Check sheet for the modelled part. Datum: model origin and axes. Units: mm. Give positions to 0.01 mm unless a question says otherwise; leave off trailing zeros. Order: outer loops, then holes, each group sorted by start corner. A loop starts at its lowest first (then second) coordinate and runs counter-clockwise, first axis right, second up.
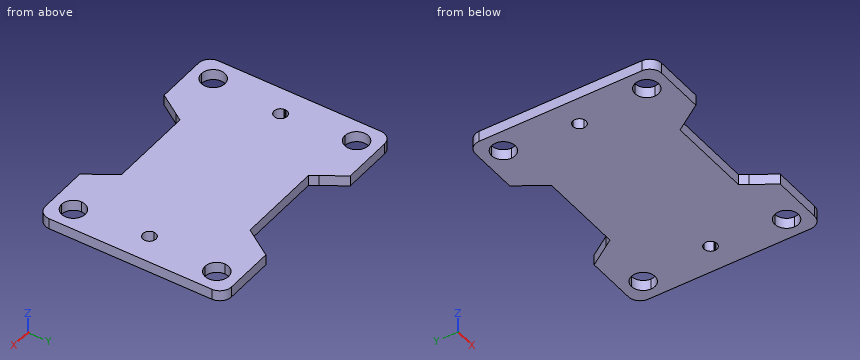
```python
from build123d import *

# Parameters (mm, degrees)
BOSS_EXTRUDE1_DEPTH = 2.5
FILLET1_R           = 2.75


with BuildPart() as part:
    # Sketch1 → Boss-Extrude1 (new body)
    with BuildSketch(Plane.XY):
        with BuildLine():
            ThreePointArc((0, 16.504235885), (-0.014991749, 16.62671172), (-0.02, 16.75))
            Line((-0.02, 16.75), (-5, 16.75))
            Line((-5, 16.75), (-5, -5))
            Line((-5, -5), (9.5, -5))
            Line((9.5, -5), (12.833333333, 0))
            Line((12.833333333, 0), (2.75, 0))
            ThreePointArc((2.75, 0), (1.944543648, -1.944543648), (0, -2.75))
            ThreePointArc((0, -2.75), (-2.75, 0), (0, 2.75))
            Line((0, 2.75), (0, 16.504235885))
        make_face()
        with BuildLine():
            ThreePointArc((0, 30.75), (-2.75, 33.5), (0, 36.25))
            ThreePointArc((0, 36.25), (1.944543648, 35.444543648), (2.75, 33.5))
            Line((2.75, 33.5), (12.833333333, 33.5))
            Line((12.833333333, 33.5), (9.5, 38.5))
            Line((9.5, 38.5), (-5, 38.5))
            Line((-5, 38.5), (-5, 16.75))
            Line((-5, 16.75), (-0.02, 16.75))
            ThreePointArc((-0.02, 16.75), (-0.014991749, 16.87328828), (0, 16.995764115))
            Line((0, 16.995764115), (0, 30.75))
        make_face()
        with BuildLine():
            ThreePointArc((2.75, 33.5), (1.944543648, 31.555456352), (0, 30.75))
            Line((0, 30.75), (0, 16.995764115))
            ThreePointArc((0, 16.995764115), (0.51591704, 17.908438918), (1.5, 18.27))
            ThreePointArc((1.5, 18.27), (2.574802307, 17.824802307), (3.02, 16.75))
            Line((3.02, 16.75), (24, 16.75))
            Line((24, 16.75), (24, 31.75))
            Line((24, 31.75), (14, 31.75))
            Line((14, 31.75), (12.833333333, 33.5))
            Line((12.833333333, 33.5), (2.75, 33.5))
        make_face()
        with BuildLine():
            Line((45.25, 33.5), (35.166666667, 33.5))
            Line((35.166666667, 33.5), (34, 31.75))
            Line((34, 31.75), (24, 31.75))
            Line((24, 31.75), (24, 16.75))
            Line((24, 16.75), (44.98, 16.75))
            ThreePointArc((44.98, 16.75), (45.425197693, 17.824802307), (46.5, 18.27))
            ThreePointArc((46.5, 18.27), (47.48408296, 17.908438918), (48, 16.995764115))
            Line((48, 16.995764115), (48, 30.75))
            ThreePointArc((48, 30.75), (46.055456352, 31.555456352), (45.25, 33.5))
        make_face()
        with BuildLine():
            Line((38.5, 38.5), (35.166666667, 33.5))
            Line((35.166666667, 33.5), (45.25, 33.5))
            ThreePointArc((45.25, 33.5), (46.055456352, 35.444543648), (48, 36.25))
            ThreePointArc((48, 36.25), (49.944543648, 35.444543648), (50.75, 33.5))
            ThreePointArc((50.75, 33.5), (49.944543648, 31.555456352), (48, 30.75))
            Line((48, 30.75), (48, 16.995764115))
            ThreePointArc((48, 16.995764115), (48.014991749, 16.87328828), (48.02, 16.75))
            Line((48.02, 16.75), (53, 16.75))
            Line((53, 16.75), (53, 38.5))
            Line((53, 38.5), (38.5, 38.5))
        make_face()
        with BuildLine():
            ThreePointArc((48.02, 16.75), (48.014991749, 16.62671172), (48, 16.504235885))
            Line((48, 16.504235885), (48, 2.75))
            ThreePointArc((48, 2.75), (49.944543648, 1.944543648), (50.75, 0))
            ThreePointArc((50.75, 0), (49.944543648, -1.944543648), (48, -2.75))
            ThreePointArc((48, -2.75), (46.055456352, -1.944543648), (45.25, 0))
            Line((45.25, 0), (35.166666667, 0))
            Line((35.166666667, 0), (38.5, -5))
            Line((38.5, -5), (53, -5))
            Line((53, -5), (53, 16.75))
            Line((53, 16.75), (48.02, 16.75))
        make_face()
        with BuildLine():
            Line((44.98, 16.75), (24, 16.75))
            Line((24, 16.75), (24, 1.75))
            Line((24, 1.75), (34, 1.75))
            Line((34, 1.75), (35.166666667, 0))
            Line((35.166666667, 0), (45.25, 0))
            ThreePointArc((45.25, 0), (46.055456352, 1.944543648), (48, 2.75))
            Line((48, 2.75), (48, 16.504235885))
            ThreePointArc((48, 16.504235885), (46.37671172, 15.235008251), (44.98, 16.75))
        make_face()
        with BuildLine():
            ThreePointArc((3.02, 16.75), (1.62328828, 15.235008251), (0, 16.504235885))
            Line((0, 16.504235885), (0, 2.75))
            ThreePointArc((0, 2.75), (1.944543648, 1.944543648), (2.75, 0))
            Line((2.75, 0), (12.833333333, 0))
            Line((12.833333333, 0), (14, 1.75))
            Line((14, 1.75), (24, 1.75))
            Line((24, 1.75), (24, 16.75))
            Line((24, 16.75), (3.02, 16.75))
        make_face()
    extrude(amount=BOSS_EXTRUDE1_DEPTH)

    # Fillet1
    fillet1_edges = [part.edges().sort_by_distance(p)[0] for p in [
        (53, -5, 1.25),
        (-5, -5, 1.25),
        (-5, 38.5, 1.25),
        (53, 38.5, 1.25),
    ]]
    fillet(fillet1_edges, radius=FILLET1_R)


solid = part.part
```
(1) Material ranges on L1, parallel to Y at x = 47.5, z = 0.9; L2, parallel to X at y = 18, z = 0.3; L3, parallel to X at y = 32, z = 0.3, recorded low to high.
Response values:
L1: y = -5 to -2.7, 2.7 to 15.61, 17.89 to 30.8, 36.2 to 38.5
L2: x = -5 to 0.64, 2.36 to 45.64, 47.36 to 53
L3: x = -5 to -2.3, 2.3 to 13.83, 34.17 to 45.7, 50.3 to 53
(2) Cross-section at C-C on z = 0.5. Enter the section's corners in (x, y), then the cut area to 3 significant figures.
Response values:
outline: (-5, -2.25) arc R2.75 ccw to (-2.25, -5) - (9.5, -5) - (14, 1.75) - (34, 1.75) - (38.5, -5) - (50.25, -5) arc R2.75 ccw to (53, -2.25) - (53, 35.75) arc R2.75 ccw to (50.25, 38.5) - (38.5, 38.5) - (34, 31.75) - (14, 31.75) - (9.5, 38.5) - (-2.25, 38.5) arc R2.75 ccw to (-5, 35.75) - close; hole circle Ø5.5 at (0, 0); hole circle Ø5.5 at (0, 33.5); hole circle Ø3.04 at (1.5, 16.75); hole circle Ø3.04 at (46.5, 16.75); hole circle Ø5.5 at (48, 0); hole circle Ø5.5 at (48, 33.5)
area: 2,080 mm2
(3) Gauge pin test, flat end, axial feed: pin 1 Ø1.2 at (x, z) = (23.5, 0.5) entering from -Y. Record the tip position at first contact, or that the pin passes through.
Response values:
pin 1: stops at y = 1.75
(4) Cross-section at A-A on x = 49. Enter the section's corners in (y, z).
Response values:
outline: (-5, 0) - (-2.56, 0) - (-2.56, 2.5) - (-5, 2.5) - close; (2.56, 0) - (30.94, 0) - (30.94, 2.5) - (2.56, 2.5) - close; (36.06, 0) - (38.5, 0) - (38.5, 2.5) - (36.06, 2.5) - close
(5) Cross-section at B-B on x = 17. Enter the section's corners in (y, z).
Response values:
outline: (1.75, 0) - (31.75, 0) - (31.75, 2.5) - (1.75, 2.5) - close
(6) Cross-section at D-D on x = 10.5. Enter the section's corners in (y, z).
Response values:
outline: (-3.5, 0) - (37, 0) - (37, 2.5) - (-3.5, 2.5) - close
